Read the model definition and answer for the solid it produces. Units are mm, in the model's axes. Face numbers are marked on the shaded views. A direction names the side the tool comes from. Give positions to 0.01 mm unless a question says otherwise; leave off trailing zeros. Loops run counter-clockwise (first coordinate to the right, second up) from the corner with the lowest first, then second, coordinate; pieces in that order, holes last.
(1) Find section A-A, the plane z = 34. Write down the section's boundary in (x, y).
(2) Each of these flat-tipped pins is pushed along its axis until it touches: P1, Ø6.5, axis at x = 15.5, y = -15.5, coming from the -Z side; P2, Ø2.5, axis at x = -15.5, y = 15.5, coming from the -Z side; P3, Ø6.5, axis at x = -16, y = 16, coming from the +Z side; P4, Ø1, axis at y = 14.5, z = 21, coming from the -X side (3 decimals). Where does it stop, or does it pass through?
(3) Straight lines are drawn through the part: probe 1 along Y at (x, z) = (15.5, 4.5); probe 2 along X at (y, z) = (15, 6); probe 3 along Z at (x, y) = (-10, 1). For each, find the intervals that lie inside material, in ascending order.
(4) Which of the six approach directions +Z, -Z, +X, -X, +Y, -Y give full straight-line access (tool end or side, diameter ignored) to the marked faces 1, 2, 3 and 4?
(5) Find section D-D, the plane y = 0. Write down the section's boundary in (x, z), then the cut area to 3 significant figures.
(6) Find section B-B, the plane x = -15.5. Write down the section's boundary in (y, z).
```python
from build123d import *

# Parameters (mm, degrees)
SKETCH1_W           = 38
SKETCH1_H           = 38
BOSS_EXTRUDE1_DEPTH = 10
SKETCH2_R           = 2
CUT_EXTRUDE1_DEPTH  = 29.670542374
BOSS_EXTRUDE2_DEPTH = 30
SKETCH8_R           = 2.5
BOSS_EXTRUDE4_DEPTH = 10


with BuildPart() as part:
    # Sketch1 → Boss-Extrude1 (new body)
    with BuildSketch(Plane.XY):
        Rectangle(SKETCH1_W, SKETCH1_H)
    extrude(amount=BOSS_EXTRUDE1_DEPTH)

    # Sketch2 → Cut-Extrude1 (cut, through all)
    with BuildSketch(Plane.XY.offset(10)):
        with Locations((15.5, 15.5)):
            Circle(SKETCH2_R)
        with Locations((15.5, -15.5)):
            Circle(SKETCH2_R)
        with Locations((-15.5, -15.5)):
            Circle(SKETCH2_R)
        with Locations((-15.5, 15.5)):
            Circle(SKETCH2_R)
    extrude(amount=-CUT_EXTRUDE1_DEPTH, mode=Mode.SUBTRACT)

    # Sketch6 → Boss-Extrude2 (add)
    with BuildSketch(Plane.XY.offset(10)):
        with BuildLine():
            Line((-19, 11), (-19, -11))
            ThreePointArc((-19, -11), (-13.343145751, -13.343145751), (-11, -19))
            Line((-11, -19), (11, -19))
            ThreePointArc((11, -19), (13.343145751, -13.343145751), (19, -11))
            Line((19, -11), (19, 11))
            ThreePointArc((19, 11), (13.343145751, 13.343145751), (11, 19))
            Line((11, 19), (-11, 19))
            ThreePointArc((-11, 19), (-13.343145751, 13.343145751), (-19, 11))
        make_face()
    extrude(amount=BOSS_EXTRUDE2_DEPTH)

    # Sketch8 → Boss-Extrude4 (add)
    with BuildSketch(Plane(origin=(0, 0, 0), x_dir=(-1, 0, 0), z_dir=(0, 0, -1))):
        Circle(SKETCH8_R)
    extrude(amount=BOSS_EXTRUDE4_DEPTH)


solid = part.part
```
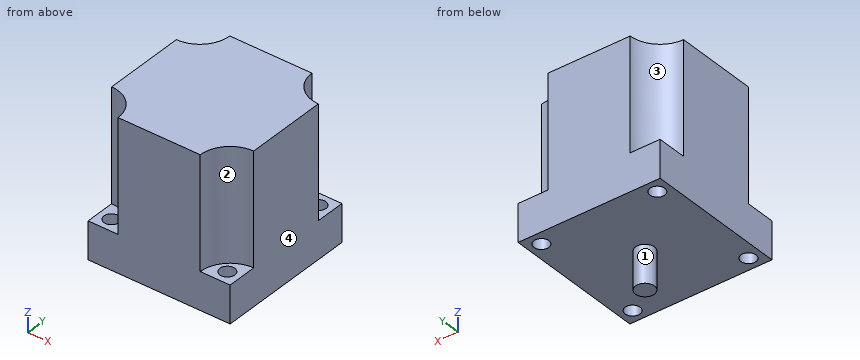
Entries:
1. outline: (-19, -11) arc R8 cw to (-11, -19) - (11, -19) arc R8 cw to (19, -11) - (19, 11) arc R8 cw to (11, 19) - (-11, 19) arc R8 cw to (-19, 11) - close
2. P1: stops at z = 0
2. P2: passes through
2. P3: stops at z = 10
2. P4: stops at x = -12.755
3. probe 1: y = -19 to -17.5, -13.5 to 13.5, 17.5 to 19
3. probe 2: x = -19 to -17.44, -13.56 to 13.56, 17.44 to 19
3. probe 3: z = 0 to 40
4. face 1: -Z
4. face 2: +Z, +X, -Y
4. face 3: +Z, -X, +Y
4. face 4: +Z, -Z, +X, +Y, -Y
5. outline: (-19, 0) - (-2.5, 0) - (-2.5, -10) - (2.5, -10) - (2.5, 0) - (19, 0) - (19, 40) - (-19, 40) - close
5. area: 1,570 mm2
6. outline: (-19, 0) - (-17.5, 0) - (-17.5, 10) - (-19, 10) - close; (-13.5, 0) - (13.5, 0) - (13.5, 10) - (11.81, 10) - (11.81, 40) - (-11.81, 40) - (-11.81, 10) - (-13.5, 10) - close; (17.5, 0) - (19, 0) - (19, 10) - (17.5, 10) - close
